Design review of the part built by this model. Coordinates are the model's own, in mm. Give positions to 0.01 mm unless a question says otherwise; leave off trailing zeros. Order: outer loops, then holes, each group sorted by start corner. A loop starts at its lowest first (then second) coordinate and runs counter-clockwise, first axis right, second up.
Autodesk Inventor part; units mm, degrees
ref_plane "YZ Plane" through (0, 0, 0) normal (1, 0, 0) x (0, 1, 0)
ref_plane "XZ Plane" through (0, 0, 0) normal (0, 1, 0) x (-1, 0, 0)
ref_plane "XY Plane" through (0, 0, 0) normal (0, 0, 1) x (1, 0, 0)
sketch "Esboço1" plane through (0, 0, 0) normal (1, 0, 0) x (0, 1, 0)
  line L0 (-129, 129) -> (129, 129)
  line L1 (129, 129) -> (129, -129)
  line L2 (129, -129) -> (-129, -129)
  line L3 (-129, -129) -> (-129, 129)
  line L4 (-129, 129) -> (129, -129) construction
  line L5 (129, 129) -> (-129, -129) construction
  point P0 (0, 0)
  dimension "d0" = 258
  dimension "d1" = 258
extrude "Extrusão1" add sketch "Esboço1" along normal mid plane 4
sketch "Esboço2" plane through (2, 0, 0) normal (1, 0, 0) x (0, 0, -1)
  line L0 (129, 129) -> (-129, 129)
  line L1 (-129, 129) -> (-41.5, 129)
  line L2 (-41.5, 129) -> (-41.5, 125)
  line L3 (-41.5, 125) -> (-129, 125)
  line L4 (-129, 125) -> (-129, 129)
  line L5 (129, 129) -> (41.5, 129)
  line L6 (41.5, 129) -> (41.5, 125)
  line L7 (41.5, 125) -> (129, 125)
  line L8 (129, 125) -> (129, 129)
  line L9 (-129, 129) -> (-129, -129)
  line L10 (-129, -129) -> (-41.5, -129)
  line L11 (-41.5, -129) -> (-41.5, -125)
  line L12 (-41.5, -125) -> (-129, -125)
  line L13 (-129, -125) -> (-129, -129)
  line L14 (129, -129) -> (129, 129)
  line L15 (129, -129) -> (41.5, -129)
  line L16 (41.5, -129) -> (41.5, -125)
  line L17 (41.5, -125) -> (129, -125)
  line L18 (129, -125) -> (129, -129)
  point P0 (0, 0)
  point P1 (129, -125)
  dimension "d4" = 87.5
  dimension "d5" = 4
  dimension "d6" = 87.5
  dimension "d7" = 4
  dimension "d8" = 83
  dimension "d9" = 87.5
  dimension "d10" = 4
  dimension "d11" = 87.5
  dimension "d12" = 4
  dimension "d13" = 83
extrude "Extrusão2" cut sketch "Esboço2" along normal through all both and the other way through all
sketch "Esboço3" plane through (2, 0, 0) normal (1, 0, 0) x (0, 0, -1)
  line L0 (-125, 41.5) -> (-133, 41.5)
  line L1 (-133, 41.5) -> (-133, -41.5)
  line L2 (-133, -41.5) -> (-125, -41.5)
  line L3 (-125, -41.5) -> (-125, 41.5)
  line L4 (-129, -125) -> (-129, 125)
  line L5 (-125, 41.5) -> (-133, -41.5) construction
  line L6 (-133, 41.5) -> (-125, -41.5) construction
  line L7 (125, -41.5) -> (133, -41.5)
  line L8 (133, -41.5) -> (133, 41.5)
  line L9 (133, 41.5) -> (125, 41.5)
  line L10 (125, 41.5) -> (125, -41.5)
  line L11 (129, 125) -> (129, -125)
  line L12 (125, -41.5) -> (133, 41.5) construction
  line L13 (133, -41.5) -> (125, 41.5) construction
  line L14 (-41.5, 125) -> (-129, 125)
  line L15 (-129, -125) -> (-41.5, -125)
  line L16 (129, 125) -> (41.5, 125)
  line L17 (41.5, -125) -> (129, -125)
  point P0 (0, 0)
  point P1 (-129, 0)
  point P2 (129, 0)
  dimension "d16" = 83
  dimension "d17" = 8
  dimension "d18" = 8
  dimension "d19" = 83
  dimension "d20" = 83.5
  dimension "d21" = 83.5
  dimension "d22" = 83.5
  dimension "d23" = 83.5
extrude "Extrusão3" cut sketch "Esboço3" along normal through all both and the other way through all
sketch "Esboço4" plane through (2, 0, 0) normal (1, 0, 0) x (0, 0, -1)
  point P0 (0, 0)
properties part number "FUNDO POÇO"
1. For line 1 along Z through (x, y) = (1, -5), list the stretches that pass through material, from the lowest coordinate up.
Recorded:
line 1: z = -125 to 125
2. Take a section at A-A (x = -0.55). State the section outline as (y, z) points.
Recorded:
outline: (-129, -41.5) - (-125, -41.5) - (-125, -129) - (-41.5, -129) - (-41.5, -125) - (41.5, -125) - (41.5, -129) - (125, -129) - (125, -41.5) - (129, -41.5) - (129, 41.5) - (125, 41.5) - (125, 129) - (41.5, 129) - (41.5, 125) - (-41.5, 125) - (-41.5, 129) - (-125, 129) - (-125, 41.5) - (-129, 41.5) - close
3. Take a section at B-B (z = 74). State the section outline as (x, y) points.
Recorded:
outline: (-2, -125) - (2, -125) - (2, 125) - (-2, 125) - close
4. For pin 1 (2 mm diameter, centred on x = 1, z = -96.5, fed in from -Y); pin 2 (1.2 mm diameter, centred on x = 0, y = 126, fed in from -Z); pin 3 (1.2 mm diameter, centred on x = -0.5, z = 126, fed in from +Y), all flat-tipped, find the tip position at first contact; note any pin that passes through.
Recorded:
pin 1: stops at y = -125
pin 2: stops at z = -41.5
pin 3: stops at y = 125
